Can you work these out from the model? Positions are in its coordinate system, mm. Face numbers are marked on the shaded views. A direction names the side the tool comes from. Give positions to 0.01 mm unless a question says otherwise; leave off trailing zeros. Order: outer loops, then holes, each group sorted by start corner. A loop starts at its lowest first (then second) coordinate and runs counter-clockwise, first axis right, second up. Notation, with made-up numbers: (75, 14.25) - (106, 14.25) arc R15 cw to (106, 21.25) - close; hole circle Ø11 at (-36.5, -7). An arc over 180 degrees is marked (long way). Answer as a JSON object with one key per item and string values.
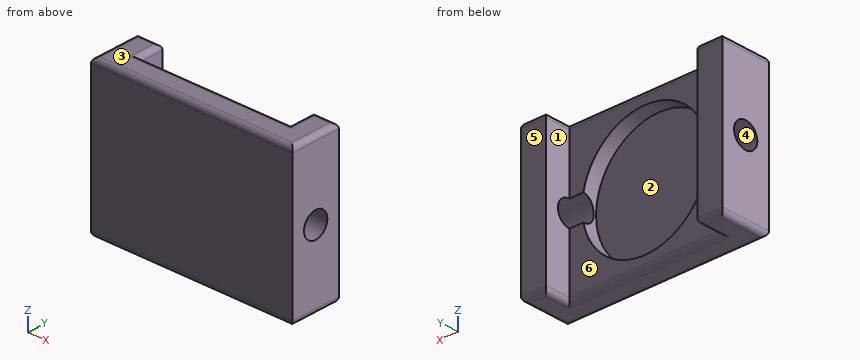
```python
from build123d import *

# Parameters (mm, degrees)
SKETCH_1_W          = 40
SKETCH_1_H          = 30
EXTRUDE_1_DEPTH     = 10
SKETCH_3_R          = 2.5
CUT_EXTRUDE_1_DEPTH = 51.990195136
CUT_EXTRUDE_2_DEPTH = 5
SKETCH_5_R          = 12.5
CUT_EXTRUDE_3_DEPTH = 3
FILLET_1_R          = 1


with BuildPart() as part:
    # 草图1 → 凸台-拉伸1 (new body)
    with BuildSketch(Plane(origin=(0, 0, 0), x_dir=(1, 0, 0), z_dir=(0, 1, 0))):
        with Locations((20, 15)):
            Rectangle(SKETCH_1_W, SKETCH_1_H)
    extrude(amount=EXTRUDE_1_DEPTH)

    # 草图3 → 切除-拉伸1 (cut, through all)
    with BuildSketch(Plane.ZY):
        with Locations((-15, 5)):
            Circle(SKETCH_3_R)
    extrude(amount=-CUT_EXTRUDE_1_DEPTH, mode=Mode.SUBTRACT)

    # 草图4 → 切除-拉伸2 (cut)
    with BuildSketch(Plane(origin=(0, 10, 0), x_dir=(1, 0, 0), z_dir=(0, 1, 0))):
        Polygon((20, 30), (5, 30), (5, 0), (35, 0), (35, 30), align=None)
    extrude(amount=-CUT_EXTRUDE_2_DEPTH, mode=Mode.SUBTRACT)

    # 草图5 → 切除-拉伸3 (cut)
    with BuildSketch(Plane(origin=(0, 5, 0), x_dir=(1, 0, 0), z_dir=(0, 1, 0))):
        with Locations(Location((20, 15, 0), (0, 0, 270))):
            Circle(SKETCH_5_R)
    extrude(amount=-CUT_EXTRUDE_3_DEPTH, mode=Mode.SUBTRACT)

    # 圆角1
    fillet_1_edges = [part.edges().sort_by_distance(p)[0] for p in [
        (37.5, 10, -30),
        (37.5, 10, 0),
        (2.5, 10, -30),
        (35, 7.5, -30),
        (5, 7.5, 0),
        (20, 5, 0),
        (35, 7.5, 0),
        (20, 5, -30),
        (5, 7.5, -30),
        (20, 0, -30),
        (20, 0, 0),
        (2.5, 10, 0),
        (0, 5, -30),
        (40, 5, -30),
        (40, 5, 0),
        (0, 5, 0),
    ]]
    fillet(fillet_1_edges, radius=FILLET_1_R)


solid = part.part
```
Q1. I need wall thicknesses on L1, parallel to X at y = 8.25, z = -23.5; L2, parallel to Y at x = 3, z = -15; L3, parallel to Z at x = 37.5, y = 5. Which ranges of each line are inside material? Lowest first, please.
Recorded:
{"L1": "x = 0 to 5, 35 to 40", "L2": "y = 0 to 2.5, 7.5 to 10", "L3": "z = -30 to -17.5, -12.5 to 0"}
Q2. I'm going to push flat-ended pins straight in: pin 1 Ø3 at (y, z) = (5, -15) entering from +X; pin 2 Ø3 at (x, z) = (21.5, -20.5) entering from +Y; pin 3 Ø4 at (x, z) = (7.5, -26.5) entering from +Y. Where does each tip first touch, or does it pass through?
Recorded:
{"pin 1": "passes through", "pin 2": "stops at y = 2", "pin 3": "stops at y = 5"}
Q3. If we section it at B-B, the plane z = -22.5: Please give me the cut outline in (x, y), then the cut area to 3 significant figures.
Recorded:
{"outline": "(0, 0) - (40, 0) - (40, 10) - (35, 10) - (35, 5) - (30, 5) - (30, 2) - (10, 2) - (10, 5) - (5, 5) - (5, 10) - (0, 10) - close", "area": "190 mm^2"}
Q4. We'd pull the mould along Z, two halves only. Please class the marked faces 1, 2, 3 and 4: released by +Z, released by -Z, zero draft, split by the parting line, or undercut.
Recorded:
{"face 1": "zero draft", "face 2": "undercut", "face 3": "released by +Z", "face 4": "undercut"}
Q5. Which directions (+Z, -Z, +X, -X, +Y, -Y) give clear straight access to the entire face, cutting with the end or side of a thin tool? Please do the marked faces 5 and 6.
Recorded:
{"face 5": "+Z, -Z, +X, -X, +Y", "face 6": "+Z, -Z, +Y"}
Q6. If we section it at A-A, the plane y = 8.25: Please give me the cut outline in (x, z), then the cut area to 3 significant figures.
Recorded:
{"outline": "(0, -29) arc R1 ccw to (1, -30) - (4, -30) arc R1 ccw to (5, -29) - (5, -1) arc R1 ccw to (4, 0) - (1, 0) arc R1 ccw to (0, -1) - close; (35, -29) arc R1 ccw to (36, -30) - (39, -30) arc R1 ccw to (40, -29) - (40, -1) arc R1 ccw to (39, 0) - (36, 0) arc R1 ccw to (35, -1) - close", "area": "298 mm^2"}
Q7. If we section it at D-D, the plane x = 20: Please give me the cut outline in (y, z).
Recorded:
{"outline": "(0, -29) arc R1 ccw to (1, -30) - (4, -30) arc R1 ccw to (5, -29) - (5, -27.5) - (2, -27.5) - (2, -2.5) - (5, -2.5) - (5, -1) arc R1 ccw to (4, 0) - (1, 0) arc R1 ccw to (0, -1) - close"}
Q8. If we section it at C-C, the plane z = -15: Please give me the cut outline in (x, y).
Recorded:
{"outline": "(0, 0) - (40, 0) - (40, 2.5) - (32.5, 2.5) - (32.5, 2) - (7.5, 2) - (7.5, 2.5) - (0, 2.5) - close; (0, 7.5) - (5, 7.5) - (5, 10) - (0, 10) - close; (35, 7.5) - (40, 7.5) - (40, 10) - (35, 10) - close"}
